Read the model definition and answer for the solid it produces. Units are mm, in the model's axes. A direction names the side the tool comes from. Coordinates: 2 decimals unless noted, no trailing zeros. Write each loop counter-clockwise with the first axis right and the second up, starting at its lowest first coordinate (ties: lowest second). Pieces come first, ordered by that corner, then holes.
Item 1: Straight lines are drawn through the part: probe 1 along Z at (x, y) = (-15.5, -6.8); probe 2 along Z at (x, y) = (-15.5, -6.1); probe 3 along X at (y, z) = (-37, -1). For each, find the intervals that lie inside material, in ascending order.
Item 2: Each of these flat-tipped pins is pushed along its axis until it touches: P1, Ø4.5, axis at x = -12.5, y = -37.5, coming from the +Z side; P2, Ø5.5, axis at x = 15.5, z = 47.93, coming from the +Y side. Where does it stop, or does it pass through?
Item 3: Determine the mould class of faces 3 (the face through (0, -7, 53.433)), 4 (the face through (-15.88, -6.51, 49.64)), 5 (the face through (-23.5, -46.07, -0.99)), 6 (the face through (-0.35, -6.073, -1.396)) for opening direction Z: released by +Z, released by -Z, zero draft, split by the parting line, or undercut.
Item 4: A tool of negligible diameter and unlimited length cuts with its end or side. For faces 1 (the face through (0, -27, 0)), 2 (the face through (-15.73, -6.51, 15.2)), from which of +Z, -Z, +X, -X, +Y, -Y can it reach the whole face along a straight path? Write none if from no direction.
Item 5: Section C-C (z = 37) is taken. Give the vertices of the cut face in (x, y), then the cut area to 3 significant figures.
Item 6: Section A-A (y = -37.5) is taken. Give the vertices of the cut face in (x, z).
from build123d import *

# Parameters (mm, degrees)
SCHIZZO1_R                             = 1.75
SCHIZZO1_R_2                           = 11.05
SCHIZZO1_R_3                           = 2
BASE_FLANGIA1_DEPTH                    = 2
PIEGATURA_START                        = -5.5
PIEGATURA_DELLO_SCHIZZO1_OUTLINE_W     = 50
PIEGATURA_DELLO_SCHIZZO1_OUTLINE_H     = 2
PIEGATURA_DELLO_SCHIZZO1_DEPTH         = 53
PIEGATURA_START_2                      = -7.5
PIEGATURA_DELLO_SCHIZZO1_2_OUTLINE_R   = 1.75
PIEGATURA_DELLO_SCHIZZO1_2_OUTLINE_R_2 = 11.05
PIEGATURA_DELLO_SCHIZZO1_2_DEPTH       = 2
PIEGATURA_START_3                      = -26
PIEGATURA_DELLO_SCHIZZO1_3_DEPTH       = 52
PIEGATURA_START_4                      = -25
PIEGATURA_DELLO_SCHIZZO1_4_DEPTH       = 50


with BuildPart() as part:
    # Base-Flangia1: sheet metal written as solids
    # Schizzo1 → Base-Flangia1 (new body)
    with BuildSketch(Plane.XY):
        with BuildLine():
            Line((-25, 42.5), (-20, 47.5))
            Line((-20, 47.5), (20, 47.5))
            Line((20, 47.5), (25, 42.5))
            Line((25, 42.5), (25, -42.5))
            ThreePointArc((25, -42.5), (23.535533906, -46.035533906), (20, -47.5))
            Line((20, -47.5), (-20, -47.5))
            ThreePointArc((-20, -47.5), (-23.535533906, -46.035533906), (-25, -42.5))
            Line((-25, -42.5), (-25, 42.5))
        make_face()
        with Locations((-15.5, 42)):
            Circle(SCHIZZO1_R, mode=Mode.SUBTRACT)
        with Locations((15.5, 42)):
            Circle(SCHIZZO1_R, mode=Mode.SUBTRACT)
        with Locations((15.5, 11)):
            Circle(SCHIZZO1_R, mode=Mode.SUBTRACT)
        with Locations((-15.5, 11)):
            Circle(SCHIZZO1_R, mode=Mode.SUBTRACT)
        with Locations((0, 26.5)):
            Circle(SCHIZZO1_R_2, mode=Mode.SUBTRACT)
        with Locations((-12.5, -37.5)):
            Circle(SCHIZZO1_R_3, mode=Mode.SUBTRACT)
        with Locations((12.5, -37.5)):
            Circle(SCHIZZO1_R_3, mode=Mode.SUBTRACT)
    extrude(amount=-BASE_FLANGIA1_DEPTH)

    # Piegatura dello schizzo1: read off the stored shape, not the designer's step
    # Piegatura dello schizzo1 outline → Piegatura dello schizzo1 (cut)
    with BuildSketch(Plane(origin=(0, 0, 0), x_dir=(1, 0, 0), z_dir=(0, 1, 0)).offset(PIEGATURA_START)):
        with Locations((0, 1)):
            Rectangle(PIEGATURA_DELLO_SCHIZZO1_OUTLINE_W, PIEGATURA_DELLO_SCHIZZO1_OUTLINE_H)
    extrude(amount=PIEGATURA_DELLO_SCHIZZO1_DEPTH, mode=Mode.SUBTRACT)

    # Piegatura dello schizzo1 2 outline → Piegatura dello schizzo1 2 (add)
    with BuildSketch(Plane(origin=(0, 0, 0), x_dir=(1, 0, 0), z_dir=(0, 1, 0)).offset(PIEGATURA_START_2)):
        Polygon((-25, 0), (-25, -48.43349571), (-20, -53.43349571), (20, -53.43349571), (25, -48.43349571), (25, 0), align=None)
        with Locations((-15.5, -47.93349571)):
            Circle(PIEGATURA_DELLO_SCHIZZO1_2_OUTLINE_R, mode=Mode.SUBTRACT)
        with Locations((15.5, -47.93349571)):
            Circle(PIEGATURA_DELLO_SCHIZZO1_2_OUTLINE_R, mode=Mode.SUBTRACT)
        with Locations((0, -32.43349571)):
            Circle(PIEGATURA_DELLO_SCHIZZO1_2_OUTLINE_R_2, mode=Mode.SUBTRACT)
        with Locations((-15.5, -16.93349571)):
            Circle(PIEGATURA_DELLO_SCHIZZO1_2_OUTLINE_R, mode=Mode.SUBTRACT)
        with Locations((15.5, -16.93349571)):
            Circle(PIEGATURA_DELLO_SCHIZZO1_2_OUTLINE_R, mode=Mode.SUBTRACT)
    extrude(amount=PIEGATURA_DELLO_SCHIZZO1_2_DEPTH)

    # Piegatura dello schizzo1 3 outline → Piegatura dello schizzo1 3 (cut)
    with BuildSketch(Plane.YZ.offset(PIEGATURA_START_3)):
        with BuildLine():
            ThreePointArc((-5.5, 0.01), (-6.08871537, -1.41128463), (-7.51, -2))
            Line((-7.51, -2), (-5.5, -2))
            Line((-5.5, -2), (-5.5, 0.01))
        make_face()
    extrude(amount=PIEGATURA_DELLO_SCHIZZO1_3_DEPTH, mode=Mode.SUBTRACT)

    # Piegatura dello schizzo1 4 outline → Piegatura dello schizzo1 4 (add)
    with BuildSketch(Plane.YZ.offset(PIEGATURA_START_4)):
        with BuildLine():
            ThreePointArc((-7.5, 0.01), (-7.502928932, 0.002928932), (-7.51, 0))
            Line((-7.51, 0), (-7.5, 0))
            Line((-7.5, 0), (-7.5, 0.01))
        make_face()
    extrude(amount=PIEGATURA_DELLO_SCHIZZO1_4_DEPTH)


solid = part.part
Established:
1. probe 1: z = -1.87 to 15.18, 18.68 to 46.18, 49.68 to 53.43
1. probe 2: z = -1.42 to 15.18, 18.68 to 46.18, 49.68 to 53.43
1. probe 3: x = -25 to -14.44, -10.56 to 10.56, 14.44 to 25
2. P1: stops at z = 0
2. P2: stops at y = -5.5
3. face 3: released by +Z
3. face 4: undercut
3. face 5: zero draft
3. face 6: released by -Z
4. face 1: +Z, +X, -X, -Y
4. face 2: +Y, -Y
5. outline: (-25, -7.5) - (-10.06, -7.5) - (-10.06, -5.5) - (-25, -5.5) - close; (10.06, -7.5) - (25, -7.5) - (25, -5.5) - (10.06, -5.5) - close
5. area: 59.8 mm2
6. outline: (-25, -2) - (-14.5, -2) - (-14.5, 0) - (-25, 0) - close; (-10.5, -2) - (10.5, -2) - (10.5, 0) - (-10.5, 0) - close; (14.5, -2) - (25, -2) - (25, 0) - (14.5, 0) - close
